Could you check a few things on this model? Use its own coordinates, in mm. A direction names the side the tool comes from. Coordinates: 2 decimals unless noted, no trailing zeros. Loops run counter-clockwise (first coordinate to the right, second up) from the corner with the lowest first, then second, coordinate; pieces in that order, holes last. Notation, with made-up numbers: (83.5, -33) - (111.5, -33) arc R38 cw to (111.5, 6) - close; hole circle Ø8 at (-12.5, 68.25). An arc over 180 degrees is marked (long way). One line per item, written item: value. Start each with the question number.
(1) If we section it at C-C on z = -6.75: Write out the boundary of the cut face in (x, y).
(2) If we section it at D-D on x = -6: Write out the boundary of the cut face in (y, z).
(3) If we mould it in two halves opening along Y, with no side actions, what happens to faces 4 (the face through (-11.5, 0, 3)), 5 (the face through (-13, 0, 1)), 6 (the face through (0, -6, -4))? For each: pulls with the +Y half, pulls with the -Y half, needs draft (parallel to the pull), parting line crosses it, or undercut.
(4) If I drill on line 1 along Y through (x, z) = (5.5, 9.9); line 2 along X through (y, z) = (3.25, -13); line 3 along Y through (x, z) = (-14, 0.85), over which ranges is the centre line in solid material (lowest first)? Write a range as from..to.
(5) On a 3-axis mill with a long thin cutter (end or side, diameter ignored), from which of +Z, -Z, +X, -X, +Y, -Y can I reach the whole of each face in a straight line? I mean faces 1 (the face through (-3.1, -0.1, 7.5)), 2 (the face through (7.885, 0.751, 10.831)), 3 (the face through (-11.5, 0, -7)). Say none if no direction works.
(6) I'm going to push flat-ended pins straight in: P1, Ø2.5, axis at x = 13, y = 1, coming from the -Z side; P2, Ø3, axis at x = 14, y = 0, coming from the +Z side; P3, Ø5, axis at x = 8.5, y = 2, coming from the +Z side; P4, Ø4.5, axis at y = 0.5, z = 4, coming from the +X side. Where does each tip first touch, or does it pass through?
(7) If we section it at B-B on y = 3.5: Write out the boundary of the cut face in (x, z), then the cut area to 3 significant figures.
(8) If we section it at A-A on x = 14: Write out the boundary of the cut face in (y, z).
```python
from build123d import *

# Parameters (mm, degrees)
SKETCH_1_W          = 32.8
SKETCH_1_H          = 12
EXTRUDE_1_DEPTH     = 1.5
SKETCH_2_W          = 23
SKETCH_2_H          = 12
EXTRUDE_2_DEPTH     = 4
SKETCH_6_W          = 23
SKETCH_6_H          = 12
EXTRUDE_5_DEPTH     = 14.5
SKETCH_7_R          = 1
CUT_EXTRUDE_2_DEPTH = 2
EXTRUDE_6_DEPTH     = 4
SKETCH_8_R          = 2.5
EXTRUDE_7_DEPTH     = 3
FILLET_1_R          = 0.3
SKETCH_9_R          = 0.75
CUT_EXTRUDE_3_DEPTH = 5
FILLET_2_R          = 0.5


with BuildPart() as part:
    # 草图1 → 凸台-拉伸1 (new body)
    with BuildSketch(Plane.XY):
        Rectangle(SKETCH_1_W, SKETCH_1_H)
    extrude(amount=EXTRUDE_1_DEPTH)

    # 草图2 → 凸台-拉伸2 (add)
    with BuildSketch(Plane.XY.offset(1.5)):
        Rectangle(SKETCH_2_W, SKETCH_2_H)
    extrude(amount=EXTRUDE_2_DEPTH)

    # 草图6 → 凸台-拉伸5 (add)
    with BuildSketch(Plane(origin=(0, 0, 0), x_dir=(-1, 0, 0), z_dir=(0, 0, -1))):
        Rectangle(SKETCH_6_W, SKETCH_6_H)
    extrude(amount=EXTRUDE_5_DEPTH)

    # 草图7 → 切除-拉伸2 (cut)
    with BuildSketch(Plane.XY.offset(1.5)):
        with Locations((-14, 0)):
            Circle(SKETCH_7_R)
        with Locations((14, 0)):
            Circle(SKETCH_7_R)
    extrude(amount=-CUT_EXTRUDE_2_DEPTH, mode=Mode.SUBTRACT)

    # 草图3 → 凸台-拉伸6 (add)
    with BuildSketch(Plane.XY.offset(5.5)):
        with BuildLine():
            Line((-0.5, 2.6), (0.092597666, 2.6))
            ThreePointArc((0.092597666, 2.6), (11.5, 0), (0.092597666, -2.6))
            Line((0.092597666, -2.6), (-0.5, -2.6))
            ThreePointArc((-0.5, -2.6), (-3.1, 0), (-0.5, 2.6))
        make_face()
    extrude(amount=EXTRUDE_6_DEPTH)

    # 草图8 → 凸台-拉伸7 (add)
    with BuildSketch(Plane.XY.offset(9.5)):
        with Locations((5.5, 0)):
            Circle(SKETCH_8_R)
    extrude(amount=EXTRUDE_7_DEPTH)

    # 圆角1
    fillet_1_edges = [part.edges().sort_by_distance(p)[0] for p in [
        (3, 0, 12.5),
    ]]
    fillet(fillet_1_edges, radius=FILLET_1_R)

    # 草图9 → 切除-拉伸3 (cut)
    with BuildSketch(Plane.XY.offset(12.5)):
        with Locations((5.5, 0)):
            Circle(SKETCH_9_R)
    extrude(amount=-CUT_EXTRUDE_3_DEPTH, mode=Mode.SUBTRACT)

    # 圆角2
    fillet_2_edges = [part.edges().sort_by_distance(p)[0] for p in [
        (0, -6, -14.5),
        (-11.5, 0, -14.5),
        (0, 6, -14.5),
        (11.5, 0, -14.5),
        (11.5, -6, 3.5),
        (11.5, -6, -7.25),
        (11.5, 6, -7.25),
        (-11.5, -6, -7.25),
        (-11.5, 6, -7.25),
        (11.5, 6, 3.5),
        (-11.5, -6, 3.5),
        (-11.5, 6, 3.5),
    ]]
    fillet(fillet_2_edges, radius=FILLET_2_R)


solid = part.part
```
Values:
1. outline: (-11.5, -5.5) arc R0.5 ccw to (-11, -6) - (11, -6) arc R0.5 ccw to (11.5, -5.5) - (11.5, 5.5) arc R0.5 ccw to (11, 6) - (-11, 6) arc R0.5 ccw to (-11.5, 5.5) - close
2. outline: (-6, -14) arc R0.5 ccw to (-5.5, -14.5) - (5.5, -14.5) arc R0.5 ccw to (6, -14) - (6, 5.5) - (-6, 5.5) - close
3. face 4: needs draft
3. face 5: undercut
3. face 6: pulls with the -Y half
4. line 1: y = -2.5..-0.75, 0.75..2.5
4. line 2: x = -11.5..11.5
4. line 3: y = -6..-1, 1..6
5. face 1: +Z, -X
5. face 2: +Z
5. face 3: -Z, -X, +Y, -Y
6. P1: stops at z = 0
6. P2: stops at z = 1.5
6. P3: stops at z = 12.5
6. P4: stops at x = 11.5
7. outline: (-16.4, 0) - (-11.5, 0) - (-11.5, -14) arc R0.5 ccw to (-11, -14.5) - (11, -14.5) arc R0.5 ccw to (11.5, -14) - (11.5, 0) - (16.4, 0) - (16.4, 1.5) - (11.5, 1.5) - (11.5, 5.5) - (10.37, 5.5) - (10.37, 9.5) - (0.63, 9.5) - (0.63, 5.5) - (-11.5, 5.5) - (-11.5, 1.5) - (-16.4, 1.5) - close
7. area: 514 mm2
8. outline: (-6, 0) - (-1, 0) - (-1, 1.5) - (-6, 1.5) - close; (1, 0) - (6, 0) - (6, 1.5) - (1, 1.5) - close
